Check sheet for the modelled part. Datum: model origin and axes. Units: mm. A direction names the side the tool comes from. Coordinates: 2 decimals unless noted, no trailing zeros. Order: outer loops, then holes, each group sorted by start corner. A loop starts at its lowest first (then second) coordinate and runs counter-clockwise, first axis right, second up.
from build123d import *

# Parameters (mm, degrees)
ESQUISSE1_R             = 80
BOSS_EXTRU_1_DEPTH      = 3
ESQUISSE2_W             = 55
ESQUISSE2_H             = 70
ENL_V_MAT_EXTRU_1_DEPTH = 114.176852757
D_GAGEMENT_M31_D        = 3.4
D_GAGEMENT_M31_DEPTH    = 24
D_GAGEMENT_M31_TIP      = 1.021463052
ESQUISSE11_W            = 52
ESQUISSE11_H            = 82
ESQUISSE11_W_2          = 57
ESQUISSE11_H_2          = 47
ENL_V_MAT_EXTRU_2_DEPTH = 108.628992377
ESQUISSE12_W            = 61
ESQUISSE12_H            = 51
ESQUISSE12_W_2          = 57
ESQUISSE12_H_2          = 47
BOSS_EXTRU_2_DEPTH      = 6


with BuildPart() as part:
    # Esquisse1 → Boss.-Extru.1 (new body)
    with BuildSketch(Plane(origin=(0, 0, 0), x_dir=(1, 0, 0), z_dir=(0, 1, 0))):
        with Locations(Location((0, 0, 0), (0, 0, 270))):
            Circle(ESQUISSE1_R)
    extrude(amount=BOSS_EXTRU_1_DEPTH)

    # Esquisse2 → Enlèv. mat.-Extru.1 (cut, through all)
    with BuildSketch(Plane(origin=(0, 3, 0), x_dir=(1, 0, 0), z_dir=(0, 1, 0))):
        with Locations((-80, 0)):
            Rectangle(ESQUISSE2_W, ESQUISSE2_H)
        with Locations((80, 0)):
            Rectangle(ESQUISSE2_W, ESQUISSE2_H)
    extrude(amount=-ENL_V_MAT_EXTRU_1_DEPTH, mode=Mode.SUBTRACT)

    # Dégagement M31
    with Locations(Plane(origin=(0, 3, 0), x_dir=(1, 0, 0), z_dir=(0, 1, 0))):
        with Locations((-45.483572208, -55), (46.516427792, -55), (-25, 69), (25, 69)):
            Hole(D_GAGEMENT_M31_D / 2, depth=D_GAGEMENT_M31_DEPTH)
            with Locations((0, 0, -(D_GAGEMENT_M31_DEPTH + D_GAGEMENT_M31_TIP / 2))):  # 118° drill point
                Cone(0, D_GAGEMENT_M31_D / 2, D_GAGEMENT_M31_TIP, mode=Mode.SUBTRACT)

    # Esquisse11 → Enlèv. mat.-Extru.2 (cut, through all)
    with BuildSketch(Plane(origin=(0, 3, 0), x_dir=(1, 0, 0), z_dir=(0, 1, 0))):
        with Locations((0, 25)):
            Rectangle(ESQUISSE11_W, ESQUISSE11_H)
        with Locations((0, -42.5)):
            Rectangle(ESQUISSE11_W_2, ESQUISSE11_H_2)
    extrude(amount=-ENL_V_MAT_EXTRU_2_DEPTH, mode=Mode.SUBTRACT)

    # Esquisse12 → Boss.-Extru.2 (add)
    with BuildSketch(Plane.XZ):
        with Locations((0, 42.5)):
            Rectangle(ESQUISSE12_W, ESQUISSE12_H)
        with Locations((0, 42.5)):
            Rectangle(ESQUISSE12_W_2, ESQUISSE12_H_2, mode=Mode.SUBTRACT)
    extrude(amount=BOSS_EXTRU_2_DEPTH)


solid = part.part
(1) Cross-section at A-A (y = 1.5). Enter the section's corners in (x, z), and give its area (3 significant figures).
Filled in:
outline: (-71.94, -35) arc R80 ccw to (71.94, -35) - (52.5, -35) - (52.5, 35) - (71.94, 35) arc R80 ccw to (-71.94, 35) - (-52.5, 35) - (-52.5, -35) - close; hole circle Ø3.4 at (-45.48, 55); hole (-28.5, 19) - (28.5, 19) - (28.5, 66) - (-28.5, 66) - close; hole circle Ø3.4 at (-25, -69); hole (-26, -66) - (26, -66) - (26, 16) - (-26, 16) - close; hole circle Ø3.4 at (25, -69); hole circle Ø3.4 at (46.52, 55)
area: 9,650 mm2
(2) Tool access check on faces 1 (the flat face through (0, -3, 17)), 2 (the flat face through (0, -1, 19)), 3 (the flat face through (30.5, -3, 42)), 4 (the flat face through (0, -3, 68)). Record the directions out of +Z, -Z, +X, -X, +Y, -Y that give a thin tool (end or side, any length) a straight path to the whole face; none if there is none.
Filled in:
face 1: -Z, +X, -X, -Y
face 2: +Y, -Y
face 3: +Z, -Z, +X, -Y
face 4: +Z, +X, -X, -Y
(3) Cross-section at C-C (x = 55). Enter the section's corners in (y, z).
Filled in:
outline: (0, -58.09) - (3, -58.09) - (3, -35) - (0, -35) - close; (0, 35) - (3, 35) - (3, 58.09) - (0, 58.09) - close
(4) Cross-section at D-D (x = 40.5). Enter the section's corners in (y, z).
Filled in:
outline: (0, -68.99) - (3, -68.99) - (3, 68.99) - (0, 68.99) - close
(5) Cross-section at B-B (z = -1.5). Enter the section's corners in (x, y).
Filled in:
outline: (-52.5, 0) - (-26, 0) - (-26, 3) - (-52.5, 3) - close; (26, 0) - (52.5, 0) - (52.5, 3) - (26, 3) - close
(6) Thickness scan on probe 1 along Z at (x, y) = (-25, 2.2); probe 2 along X at (y, z) = (0.9, 55); probe 3 along X at (y, z) = (1.4, -69). Record the ranges inside material, lowest first.
Filled in:
probe 1: z = -75.99 to -70.7, -67.3 to -66, 16 to 19, 66 to 75.99
probe 2: x = -58.09 to -47.18, -43.78 to -28.5, 28.5 to 44.82, 48.22 to 58.09
probe 3: x = -40.48 to -26.7, -23.3 to 23.3, 26.7 to 40.48
(7) Go/stop test with flat-tipped pins: P1, Ø0.9, axis at x = 58.5, y = 1.5, coming from the -Z side; P2, Ø2.5, axis at y = 1.5, z = -31.5, coming from the +X side; P3, Ø3.5, axis at x = 59, y = 1, coming from the +Z side. Record where each tip stops, or that it passes through.
Filled in:
P1: stops at z = -55.05
P2: stops at x = 52.5
P3: stops at z = 55.88
(8) Release check for a two-part mould opening along Z. For faces 5 (the flat face through (-30.5, -3, 42)), 6 (the flat face through (-28.5, -1, 42)), 7 (the cylindrical face through (1.25, 1.48, -79.99)) record: +Z half, -Z half, draft (parallel to the pull), parting line (faces both ways), or undercut.
Filled in:
face 5: draft
face 6: undercut
face 7: -Z half
